Source: CAD feature listing. Evaluate the final solid. Frame: model axes, mm. A direction names the side the tool comes from. Round coordinates to 2 decimals unless told otherwise and drop trailing zeros. Write each loop counter-clockwise with the first axis right and the second up, starting at its lowest first coordinate (ties: lowest second). Pieces come first, ordered by that corner, then holes.
from build123d import *

# Parameters (mm, degrees)
BOSS_EXTRUDE1_DEPTH = 2.5
SKETCH3_W           = 2.5
SKETCH3_H           = 60
BOSS_EXTRUDE2_DEPTH = 2.5
BOSS_EXTRUDE3_DEPTH = 20
SKETCH5_R           = 3.75
BOSS_EXTRUDE4_DEPTH = 5.5
SKETCH6_R           = 3.75
BOSS_EXTRUDE5_DEPTH = 5.5
SKETCH8_R           = 1.05
CUT_EXTRUDE1_DEPTH  = 2.5
SKETCH9_R           = 1.05
CUT_EXTRUDE2_DEPTH  = 2.5
SKETCH10_W          = 5
SKETCH10_H          = 7.5
BOSS_EXTRUDE6_DEPTH = 10
SKETCH11_W          = 2.5
SKETCH11_H          = 12.5
SKETCH11_W_2        = 2.2
BOSS_EXTRUDE7_DEPTH = 10
SKETCH12_R          = 1.5
CUT_EXTRUDE3_DEPTH  = 114
SKETCH14_W          = 30
SKETCH14_H          = 2.5
BOSS_EXTRUDE8_DEPTH = 10


with BuildPart() as part:
    # Sketch1 → Boss-Extrude1 (new body)
    with BuildSketch(Plane(origin=(0, 0, 0), x_dir=(1, 0, 0), z_dir=(0, 1, 0))):
        with BuildLine():
            Line((-62.5, 25), (-62.5, -25))
            ThreePointArc((-62.5, -25), (-53.127416998, -47.627416998), (-30.5, -57))
            Line((-30.5, -57), (-23.5, -57))
            Line((-23.5, -57), (-23.5, -35))
            Line((-23.5, -35), (-30.5, -35))
            ThreePointArc((-30.5, -35), (-40.5, -25), (-30.5, -15))
            Line((-30.5, -15), (38.5, -15))
            ThreePointArc((38.5, -15), (48.5, -25), (38.5, -35))
            Line((38.5, -35), (31.5, -35))
            Line((31.5, -35), (31.5, -57))
            Line((31.5, -57), (38.5, -57))
            Line((38.5, -57), (62.5, -57))
            Line((62.5, -57), (62.5, 57))
            Line((62.5, 57), (38.5, 57))
            Line((38.5, 57), (31.5, 57))
            Line((31.5, 57), (31.5, 35))
            Line((31.5, 35), (38.5, 35))
            ThreePointArc((38.5, 35), (48.5, 25), (38.5, 15))
            Line((38.5, 15), (-30.5, 15))
            ThreePointArc((-30.5, 15), (-40.5, 25), (-30.5, 35))
            Line((-30.5, 35), (-23.5, 35))
            Line((-23.5, 35), (-23.5, 57))
            Line((-23.5, 57), (-30.5, 57))
            ThreePointArc((-30.5, 57), (-53.127416998, 47.627416998), (-62.5, 25))
        make_face()
    extrude(amount=BOSS_EXTRUDE1_DEPTH)

    # Sketch3 → Boss-Extrude2 (add)
    # profile 1 of 3: a face of its own
    with BuildSketch(Plane(origin=(0, 2.5, 0), x_dir=(1, 0, 0), z_dir=(0, 1, 0))):
        with BuildLine():
            Line((-30.5, -2.5), (38.5, -2.5))
            ThreePointArc((38.5, -2.5), (61, -25), (38.5, -47.5))
            Line((38.5, -47.5), (38.5, -57))
            Line((38.5, -57), (31.5, -57))
            Line((31.5, -57), (31.5, -35))
            Line((31.5, -35), (38.5, -35))
            Line((38.5, -35), (38.5, -40))
            ThreePointArc((38.5, -40), (53.5, -25), (38.5, -10))
            Line((38.5, -10), (-30.5, -10))
            ThreePointArc((-30.5, -10), (-45.5, -25), (-30.5, -40))
            Line((-30.5, -40), (-30.5, -35))
            Line((-30.5, -35), (-23.5, -35))
            Line((-23.5, -35), (-23.5, -57))
            Line((-23.5, -57), (-30.5, -57))
            Line((-30.5, -57), (-30.5, -47.5))
            ThreePointArc((-30.5, -47.5), (-53, -25), (-30.5, -2.5))
        make_face()
        with BuildLine():
            Line((-30.5, -5), (38.5, -5))
            ThreePointArc((38.5, -5), (58.5, -25), (38.5, -45))
            Line((38.5, -45), (38.5, -42.5))
            ThreePointArc((38.5, -42.5), (56, -25), (38.5, -7.5))
            Line((38.5, -7.5), (-30.5, -7.5))
            ThreePointArc((-30.5, -7.5), (-48, -25), (-30.5, -42.5))
            Line((-30.5, -42.5), (-30.5, -45))
            ThreePointArc((-30.5, -45), (-50.5, -25), (-30.5, -5))
        make_face(mode=Mode.SUBTRACT)
    # profile 2 of 3: a face of its own
    with BuildSketch(Plane(origin=(0, 2.5, 0), x_dir=(1, 0, 0), z_dir=(0, 1, 0))):
        with Locations((-56.25, 0)):
            Rectangle(SKETCH3_W, SKETCH3_H)
    # profile 3 of 3: a face of its own
    with BuildSketch(Plane(origin=(0, 2.5, 0), x_dir=(1, 0, 0), z_dir=(0, 1, 0))):
        with BuildLine():
            Line((-30.5, 47.5), (-30.5, 57))
            Line((-30.5, 57), (-23.5, 57))
            Line((-23.5, 57), (-23.5, 35))
            Line((-23.5, 35), (-30.5, 35))
            Line((-30.5, 35), (-30.5, 40))
            ThreePointArc((-30.5, 40), (-45.5, 25), (-30.5, 10))
            Line((-30.5, 10), (38.5, 10))
            ThreePointArc((38.5, 10), (53.5, 25), (38.5, 40))
            Line((38.5, 40), (38.5, 35))
            Line((38.5, 35), (31.5, 35))
            Line((31.5, 35), (31.5, 57))
            Line((31.5, 57), (38.5, 57))
            Line((38.5, 57), (38.5, 47.5))
            ThreePointArc((38.5, 47.5), (61, 25), (38.5, 2.5))
            Line((38.5, 2.5), (-30.5, 2.5))
            ThreePointArc((-30.5, 2.5), (-53, 25), (-30.5, 47.5))
        make_face()
        with BuildLine():
            Line((-30.5, 42.5), (-30.5, 45))
            ThreePointArc((-30.5, 45), (-50.5, 25), (-30.5, 5))
            Line((-30.5, 5), (38.5, 5))
            ThreePointArc((38.5, 5), (58.5, 25), (38.5, 45))
            Line((38.5, 45), (38.5, 42.5))
            ThreePointArc((38.5, 42.5), (56, 25), (38.5, 7.5))
            Line((38.5, 7.5), (-30.5, 7.5))
            ThreePointArc((-30.5, 7.5), (-48, 25), (-30.5, 42.5))
        make_face(mode=Mode.SUBTRACT)
    extrude(amount=BOSS_EXTRUDE2_DEPTH)

    # Sketch4 → Boss-Extrude3 (add)
    with BuildSketch(Plane(origin=(0, 5, 0), x_dir=(1, 0, 0), z_dir=(0, 1, 0))):
        Polygon((-30.5, -35), (-23.5, -35), (-23.5, -57), (-30.5, -57), (-30.5, -54.5), (-26, -54.5), (-26, -37.5), (-30.5, -37.5), align=None)
        Polygon((38.5, -35), (31.5, -35), (31.5, -57), (38.5, -57), (38.5, -54.5), (34, -54.5), (34, -37.5), (38.5, -37.5), align=None)
        Polygon((38.5, 37.5), (38.5, 35), (31.5, 35), (31.5, 57), (38.5, 57), (38.5, 54.5), (34, 54.5), (34, 37.5), align=None)
        Polygon((-30.5, 37.5), (-30.5, 35), (-23.5, 35), (-23.5, 57), (-30.5, 57), (-30.5, 54.5), (-26, 54.5), (-26, 37.5), align=None)
    extrude(amount=BOSS_EXTRUDE3_DEPTH)

    # Sketch5 → Boss-Extrude4 (add)
    with BuildSketch(Plane.ZY.offset(-31.5)):
        with Locations(Location((46, 12.5, 0), (0, 0, 180))):
            Circle(SKETCH5_R)
    extrude(amount=BOSS_EXTRUDE4_DEPTH)

    # Sketch6 → Boss-Extrude5 (add)
    with BuildSketch(Plane.ZY.offset(-31.5)):
        with Locations(Location((-46, 12.5, 0), (0, 0, 180))):
            Circle(SKETCH6_R)
    extrude(amount=BOSS_EXTRUDE5_DEPTH)

    # Sketch8 → Cut-Extrude1 (cut)
    with BuildSketch(Plane(origin=(-23.5, 0, 0), x_dir=(0, 0, -1), z_dir=(1, 0, 0))):
        with Locations((-42.5, 22)):
            Circle(SKETCH8_R)
        with Locations(Location((-49.5, 22, 0), (0, 0, 180))):
            Circle(SKETCH8_R)
        with Locations((-49.5, 8)):
            Circle(SKETCH8_R)
        with Locations(Location((-42.5, 8, 0), (0, 0, 180))):
            Circle(SKETCH8_R)
    extrude(amount=-CUT_EXTRUDE1_DEPTH, mode=Mode.SUBTRACT)

    # Sketch9 → Cut-Extrude2 (cut)
    with BuildSketch(Plane(origin=(-23.5, 0, 0), x_dir=(0, 0, -1), z_dir=(1, 0, 0))):
        with Locations((49.5, 22)):
            Circle(SKETCH9_R)
        with Locations(Location((42.5, 22, 0), (0, 0, 180))):
            Circle(SKETCH9_R)
        with Locations((42.5, 8)):
            Circle(SKETCH9_R)
        with Locations(Location((49.5, 8, 0), (0, 0, 180))):
            Circle(SKETCH9_R)
    extrude(amount=-CUT_EXTRUDE2_DEPTH, mode=Mode.SUBTRACT)

    # Sketch10 → Boss-Extrude6 (add)
    with BuildSketch(Plane(origin=(0, 2.5, 0), x_dir=(1, 0, 0), z_dir=(0, 1, 0))):
        with Locations((60, 53.25)):
            Rectangle(SKETCH10_W, SKETCH10_H)
        with Locations((60, 0)):
            Rectangle(SKETCH10_W, SKETCH10_H)
        with Locations((60, -53.25)):
            Rectangle(SKETCH10_W, SKETCH10_H)
    extrude(amount=BOSS_EXTRUDE6_DEPTH)

    # Sketch11 → Boss-Extrude7 (add)
    with BuildSketch(Plane(origin=(62.5, 0, 0), x_dir=(0, 0, -1), z_dir=(1, 0, 0))):
        with Locations((55.75, 6.25)):
            Rectangle(SKETCH11_W, SKETCH11_H)
        with Locations((0, 6.25)):
            Rectangle(SKETCH11_W_2, SKETCH11_H)
        with Locations((50.75, 6.25)):
            Rectangle(SKETCH11_W, SKETCH11_H)
        with Locations((-50.75, 6.25)):
            Rectangle(SKETCH11_W, SKETCH11_H)
        with Locations((-55.75, 6.25)):
            Rectangle(SKETCH11_W, SKETCH11_H)
    extrude(amount=BOSS_EXTRUDE7_DEPTH)

    # Sketch12 → Cut-Extrude3 (cut)
    with BuildSketch(Plane(origin=(0, 0, -57), x_dir=(-1, 0, 0), z_dir=(0, 0, -1))):
        with Locations((-68.75, 9.375)):
            Circle(SKETCH12_R)
        with Locations((-68.75, 3.125)):
            Circle(SKETCH12_R)
    extrude(amount=-CUT_EXTRUDE3_DEPTH, mode=Mode.SUBTRACT)

    # Sketch14 → Boss-Extrude8 (add)
    with BuildSketch(Plane(origin=(62.5, 0, 0), x_dir=(0, 0, -1), z_dir=(1, 0, 0))):
        with Locations((-25.3, 1.25)):
            Rectangle(SKETCH14_W, SKETCH14_H)
        with Locations((25.3, 1.25)):
            Rectangle(SKETCH14_W, SKETCH14_H)
    extrude(amount=BOSS_EXTRUDE8_DEPTH)


solid = part.part
1) Section query A-A on x = -18. Return the cut outline in (y, z), then the cut area to 3 significant figures.
Taken from the geometry:
outline: (0, -15) - (2.5, -15) - (2.5, -10) - (5, -10) - (5, -7.5) - (2.5, -7.5) - (2.5, -5) - (5, -5) - (5, -2.5) - (2.5, -2.5) - (2.5, 2.5) - (5, 2.5) - (5, 5) - (2.5, 5) - (2.5, 7.5) - (5, 7.5) - (5, 10) - (2.5, 10) - (2.5, 15) - (0, 15) - close
area: 100 mm2
2) Reachability of faces 4 (the face through (65, 12.5, -55)), 5 (the face through (67, 6, 54.5)), 6 (the face through (-23.5, 12, 46)), 7 (the face through (53.496, 3.732, -24.67)) from +Z, -Z, +X, -X, +Y, -Y: full face, straight path, thin tool, end or side. Return the list, or none.
Taken from the geometry:
face 4: +Z, -Z, +X, +Y
face 5: +X, +Y, -Y
face 6: +Z, +Y, -Y
face 7: +Y
3) Pull-direction query (Y, two-part tool) for faces 1 (the face through (67.364, 8.8, -50.768)), 2 (the face through (-30.5, 14, 36)), 3 (the face through (33, 25, -46)); classes: released by +Y, released by -Y, zero draft, split by the parting line, or undercut.
Taken from the geometry:
face 1: undercut
face 2: zero draft
face 3: released by +Y
4) Contact query for flat-ended pins moving along their axis: P1, Ø12, axis at x = 42.5, z = 11.5, coming from the -Y side; P2, Ø2, axis at y = 8.5, z = 53, coming from the -X side; P3, Ø2.5, axis at y = 18.5, z = 38.5, coming from the -X side; P4, Ø1.2, axis at y = 8, z = 53.5, coming from the +X side. Output: stop coordinate, or through.
Taken from the geometry:
P1: stops at y = 0
P2: stops at x = -26
P3: stops at x = -30.5
P4: stops at x = 62.5
5) Material intervals for line 1 (Y direction, x = -25.2, z = -42.5); line 2 (Z direction, x = 13, y = 4); line 3 (X direction, y = 9, z = -49), sorted ascending.
Taken from the geometry:
line 1: y = 0 to 6.95, 9.05 to 20.95, 23.05 to 25
line 2: z = -10 to -7.5, -5 to -2.5, 2.5 to 5, 7.5 to 10
line 3: x = -26 to -23.5, 31.5 to 34
